```python
from build123d import *

# Parameters (mm, degrees)
SKETCH1_W           = 76.2
SKETCH1_H           = 19.05
BOSS_EXTRUDE1_DEPTH = 25.4
BOSS_EXTRUDE2_DEPTH = 25.4
CUT_EXTRUDE1_DEPTH  = 7.1374


with BuildPart() as part:
    # Sketch1 → Boss-Extrude1 (new body)
    with BuildSketch(Plane(origin=(0, 0, 0), x_dir=(1, 0, 0), z_dir=(0, 1, 0))):
        Rectangle(SKETCH1_W, SKETCH1_H)
    extrude(amount=BOSS_EXTRUDE1_DEPTH)

    # Sketch2 → Boss-Extrude2 (add)
    with BuildSketch(Plane(origin=(0, 0, 0), x_dir=(1, 0, 0), z_dir=(0, 1, 0))):
        with BuildLine():
            Line((-38.1, 9.525), (-11.879738537, 39.105310408))
            ThreePointArc((-11.879738537, 39.105310408), (0, 44.45), (11.879738537, 39.105310408))
            Line((11.879738537, 39.105310408), (38.1, 9.525))
            Line((38.1, 9.525), (38.1, -9.525))
            Line((38.1, -9.525), (-38.1, -9.525))
            Line((-38.1, -9.525), (-38.1, 9.525))
        make_face()
    extrude(amount=BOSS_EXTRUDE2_DEPTH)

    # Sketch3 → Cut-Extrude1 (cut)
    with BuildSketch(Plane(origin=(0, 25.4, 0), x_dir=(1, 0, 0), z_dir=(0, 1, 0))):
        with BuildLine():
            Line((-30.1625, -4.7625), (30.1625, -4.7625))
            ThreePointArc((30.1625, -4.7625), (32.40756403, -3.83256403), (33.3375, -1.5875))
            Line((33.3375, -1.5875), (33.3375, 6.513465997))
            ThreePointArc((33.3375, 6.513465997), (33.131023115, 7.639741058), (32.538447707, 8.619528078))
            Line((32.538447707, 8.619528078), (19.803029448, 22.986952515))
            ThreePointArc((19.803029448, 22.986952515), (16.937724791, 24.017951921), (14.522568117, 22.163242028))
            ThreePointArc((14.522568117, 22.163242028), (0, 12.7), (-14.522568117, 22.163242028))
            ThreePointArc((-14.522568117, 22.163242028), (-16.937724791, 24.017951921), (-19.803029448, 22.986952515))
            Line((-19.803029448, 22.986952515), (-32.538447707, 8.619528078))
            ThreePointArc((-32.538447707, 8.619528078), (-33.131023115, 7.639741058), (-33.3375, 6.513465997))
            Line((-33.3375, 6.513465997), (-33.3375, -1.5875))
            ThreePointArc((-33.3375, -1.5875), (-32.40756403, -3.83256403), (-30.1625, -4.7625))
        make_face()
    extrude(amount=-CUT_EXTRUDE1_DEPTH, mode=Mode.SUBTRACT)


solid = part.part
```
Read the model definition and answer for the solid it produces. Units are mm, in the model's axes. A direction names the side the tool comes from. Round coordinates to 2 decimals unless told otherwise and drop trailing zeros. Write each loop counter-clockwise with the first axis right and the second up, starting at its lowest first coordinate (ties: lowest second). Pieces come first, ordered by that corner, then holes. Notation, with made-up numbers: M 34.25,19 L 85.25,19 A25 cw 85.25,34 Z; hole C 14,19.25 d2. An arc over 180 degrees is marked long. One line per item, written item: value.
Q1. Straight lines are drawn through the part: line 1 (Y direction, x = 15, z = -17); line 2 (X direction, y = 24.5, z = -16); line 3 (Z direction, x = 13, y = 23.25) (1 decimal). For each, find the intervals that lie inside material, in ascending order. Write a range as [from, to].
Data:
line 1: [0, 18.26]
line 2: [-32.36, -26], [-9.69, 9.69], [26, 32.36]
line 3: [-37.8, -19.5], [4.8, 9.5]
Q2. Flat-ended cylindrical pins translate along their axes: pin 1 Ø10 at (x, y) = (-16, 21) entering from -Z; pin 2 Ø1.5 at (y, z) = (16, -26.5) entering from +X; pin 3 Ø2 at (x, y) = (13, 20.5) entering from -Z. Find the tip coordinate at first contact, or state that the pin passes through.
Data:
pin 1: z = -40.02
pin 2: x = 23.72
pin 3: z = -38.97
Q3. Find section C-C on z = 3.5. Write down the section's boundary in (x, y).
Data:
outline: M -38.1,0 L 38.1,0 L 38.1,25.4 L 32.7,25.4 L 32.7,18.26 L -32.7,18.26 L -32.7,25.4 L -38.1,25.4 Z
Q4. Which of the six approach directions +Z, -Z, +X, -X, +Y, -Y give full straight-line access (tool end or side, diameter ignored) to faces 1 (the flat face through (0, 22, 4.762)), 2 (the flat face through (1, 0, -12))?
Data:
face 1: +Y
face 2: +Z, -Z, +X, -X, -Y
Q5. Find section A-A on y = 16.25. Write down the section's boundary in (x, z) (3 decimals), plus the area to 3 significant figures.
Data:
outline: M -38.1,-9.525 L -11.88,-39.105 A15.875 ccw 11.88,-39.105 L 38.1,-9.525 L 38.1,9.525 L -38.1,9.525 Z
area: 3,020 mm2
Q6. Find section B-B on x = 6.5. Write down the section's boundary in (y, z) (1 decimal), plus the area to 3 significant figures.
Data:
outline: M 0,-43.1 L 25.4,-43.1 L 25.4,-14.1 L 18.3,-14.1 L 18.3,4.8 L 25.4,4.8 L 25.4,9.5 L 0,9.5 Z
area: 1,200 mm2
Q7. For a pull along Z with two mould halves and no side action, classify faces 3 (the flat face through (38.1, 13, 0)), 4 (the flat face through (-1, 13, 9.525)), 5 (the cylindrical face through (-16.89, 21.88, -24.01)), 6 (the cylindrical face through (16.982, 21.881, -24.024)) as +Z half, -Z half, draft (parallel to the pull), parting line (faces both ways), or undercut.
Data:
face 3: draft
face 4: +Z half
face 5: undercut
face 6: undercut
Q8. Find section D-D on z = -17. Write down the section's boundary in (x, y), plus the area to 3 significant figures.
Data:
outline: M -31.47,0 L 31.47,0 L 31.47,25.4 L 25.11,25.4 L 25.11,18.26 L 10.86,18.26 L 10.86,25.4 L -10.86,25.4 L -10.86,18.26 L -25.11,18.26 L -25.11,25.4 L -31.47,25.4 Z
area: 1,400 mm2
